```python
from build123d import *

# Parameters (mm, degrees)
F0_W     = 25.7
F0_H     = 25.7
F1_DEPTH = 80
F2_W     = 8
F2_H     = 30
F2_H_2   = 10
F3_DEPTH = 60
F4_R     = 6.25
F5_DEPTH = 25


with BuildPart() as f1:
    # F0 (on Front) → F1 (new body)
    with BuildSketch(Plane.XZ):
        with BuildLine():
            Line((-12.85, -14.85), (12.85, -14.85))
            ThreePointArc((12.85, -14.85), (14.264214, -14.264214), (14.85, -12.85))
            Line((14.85, -12.85), (14.85, 12.85))
            ThreePointArc((14.85, 12.85), (14.264214, 14.264214), (12.85, 14.85))
            Line((12.85, 14.85), (-12.85, 14.85))
            ThreePointArc((-12.85, 14.85), (-14.264214, 14.264214), (-14.85, 12.85))
            Line((-14.85, 12.85), (-14.85, -12.85))
            ThreePointArc((-14.85, -12.85), (-14.264214, -14.264214), (-12.85, -14.85))
        make_face()
        Rectangle(F0_W, F0_H, mode=Mode.SUBTRACT)
    extrude(amount=F1_DEPTH)

    # F2 (on face) → F3 (join)
    with BuildSketch(Plane.XY.offset(14.85)):
        with Locations((0, -15)):
            Rectangle(F2_W, F2_H)
        with Locations((0, 5)):
            Rectangle(F2_W, F2_H_2)
    extrude(amount=F3_DEPTH)

    # F4 (on face) → F5 (cut)
    with BuildSketch(Plane.YZ.offset(4)):
        with Locations((-10, 34.85)):
            Circle(F4_R)
        with Locations((-10, 59.85)):
            Circle(F4_R)
    extrude(amount=-F5_DEPTH, mode=Mode.SUBTRACT)


solid = f1.part
```
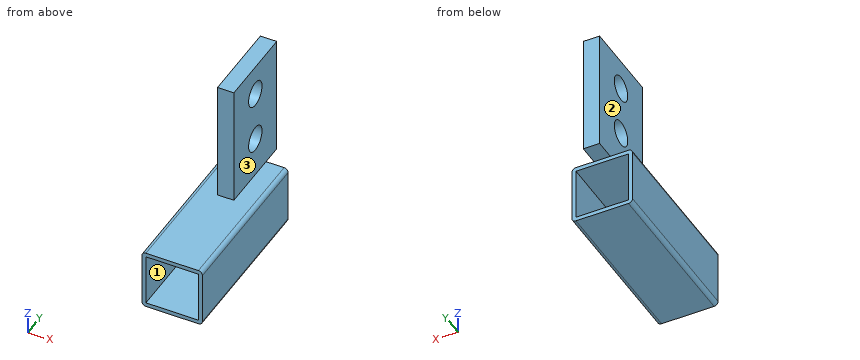
Could you check a few things on this model? Use its own coordinates, in mm. Face numbers are marked on the shaded views. A direction names the side the tool comes from. Round coordinates to 2 decimals unless told otherwise and drop trailing zeros. Loops run counter-clockwise (first coordinate to the right, second up) from the corner with the lowest first, then second, coordinate; pieces in that order, holes last. Notation, with made-up numbers: (-29, 65.25) - (10, 65.25) arc R22 cw to (10, 79.25) - close; hole circle Ø3 at (16.5, 77). An arc over 180 degrees is marked (long way). Answer in a Markdown table with one row per item. Add a question column.
(1) If we section it at B-B (z = -8): Please give me the cut outline in (x, y), plus the area to 3 significant figures.
(2) If we section it at C-C (x = 2.25): Please give me the cut outline in (y, z), plus the area to 3 significant figures.
(3) For the marked faces 1, 2 and 3, which set-ups out of +Z, -Z, +X, -X, +Y, -Y let a thin tool reach every point of the face, with its end or its side?
(4) I'm going to push flat-ended pins straight in: pin 1 (4 mm diameter, centred on x = 0, z = 48, fed in from -Y); pin 2 (1.5 mm diameter, centred on x = 8.5, y = -64, fed in from +Z); pin 3 (12 mm diameter, centred on y = -10, z = 36, fed in from +X). Where does each tip first touch, or does it pass through?
(5) If we section it at A-A (y = -10): Please give me the cut outline in (x, z).
(6) If we section it at D-D (y = -66): Please give me the cut outline in (x, z).
(7) I need wall thicknesses on line 1 along Z through (x, y) = (-1, -10); line 2 along Z through (x, y) = (-0.5, -17.5); line 3 along Z through (x, y) = (-7.75, -70). Which ranges of each line are inside material? Lowest first, please.
Model answer:
| question | item | result |
|---|---|---|
| 1 | outline | (-14.85, -80) - (-12.85, -80) - (-12.85, 0) - (-14.85, 0) - close; (12.85, -80) - (14.85, -80) - (14.85, 0) - (12.85, 0) - close |
| 1 | area | 320 mm² |
| 2 | outline | (-80, -14.85) - (0, -14.85) - (0, -12.85) - (-80, -12.85) - close; (-80, 12.85) - (0, 12.85) - (0, 14.85) - (10, 14.85) - (10, 74.85) - (-30, 74.85) - (-30, 14.85) - (-80, 14.85) - close; hole circle Ø12.5 at (-10, 34.85); hole circle Ø12.5 at (-10, 59.85) |
| 2 | area | 2,470 mm² |
| 3 | face 1 | +Y, -Y |
| 3 | face 2 | +Z, -X, +Y, -Y |
| 3 | face 3 | +Z, +X, +Y, -Y |
| 4 | pin 1 | stops at y = -30 |
| 4 | pin 2 | stops at z = 14.85 |
| 4 | pin 3 | stops at x = 4 |
| 5 | outline | (-14.85, -12.85) arc R2 ccw to (-12.85, -14.85) - (12.85, -14.85) arc R2 ccw to (14.85, -12.85) - (14.85, 12.85) arc R2 ccw to (12.85, 14.85) - (4, 14.85) - (4, 28.6) - (-4, 28.6) - (-4, 14.85) - (-12.85, 14.85) arc R2 ccw to (-14.85, 12.85) - close; (-4, 41.1) - (4, 41.1) - (4, 53.6) - (-4, 53.6) - close; (-4, 66.1) - (4, 66.1) - (4, 74.85) - (-4, 74.85) - close; hole (-12.85, -12.85) - (12.85, -12.85) - (12.85, 12.85) - (-12.85, 12.85) - close |
| 6 | outline | (-14.85, -12.85) arc R2 ccw to (-12.85, -14.85) - (12.85, -14.85) arc R2 ccw to (14.85, -12.85) - (14.85, 12.85) arc R2 ccw to (12.85, 14.85) - (-12.85, 14.85) arc R2 ccw to (-14.85, 12.85) - close; hole (-12.85, -12.85) - (12.85, -12.85) - (12.85, 12.85) - (-12.85, 12.85) - close |
| 7 | line 1 | z = -14.85 to -12.85, 12.85 to 28.6, 41.1 to 53.6, 66.1 to 74.85 |
| 7 | line 2 | z = -14.85 to -12.85, 12.85 to 74.85 |
| 7 | line 3 | z = -14.85 to -12.85, 12.85 to 14.85 |
